from build123d import *

# Parameters (mm, degrees)
F1_W     = 12
F1_H     = 2
F3_R     = 10
F5_DEPTH = 12.001
F6_R     = 2.5
F7_DEPTH = 12.001
F8_R     = 5.99999
F9_R     = 5.99999


# Not quite as in the source:
# - a fillet or chamfer is up to 0.001 mm smaller than in the source, because OpenCascade refuses the exact size


with BuildPart() as f2:
    # F2: sweep along a path in F0
    with BuildLine(Plane.YZ) as f2_path:
        Line((0, 0), (20, 0))
        Line((20, 0), (35, 10))
        Line((35, 10), (92, 10))
    # F1 (on Front) → F2 (sweep)
    with BuildSketch(Plane.XZ):
        with Locations((0, 1)):
            Rectangle(F1_W, F1_H)
    sweep(path=f2_path.line, transition=Transition.RIGHT)

    # F3
    f3_edges = [f2.edges().sort_by_distance(p)[0] for p in [
        (0, 19.394449, 2),
        (0, 34.394449, 12),
        (0, 35, 10),
        (0, 20, 0),
    ]]
    fillet(f3_edges, radius=F3_R)

    # F4 (on Top) → F5 (cut, through all)
    with BuildSketch(Plane.XY):
        with BuildLine():
            Line((2, 4.5), (2, 7.5))
            ThreePointArc((2, 7.5), (0, 8.5), (-2, 7.5))
            Line((-2, 7.5), (-2, 4.5))
            ThreePointArc((-2, 4.5), (0, 3.5), (2, 4.5))
        make_face()
    extrude(amount=F5_DEPTH, mode=Mode.SUBTRACT)

    # F6 (on Top) → F7 (cut, through all)
    with BuildSketch(Plane.XY):
        with Locations((0, 86)):
            Circle(F6_R)
    extrude(amount=F7_DEPTH, mode=Mode.SUBTRACT)

    # F8 (radius 6 in the source; OpenCascade refuses exactly that, so slightly less here)
    f8_edges = [f2.edges().sort_by_distance(p)[0] for p in [
        (-6, 0, 1),
        (6, 0, 1),
    ]]
    fillet(f8_edges, radius=F8_R)

    # F9 (radius 6 in the source; OpenCascade refuses exactly that, so slightly less here)
    f9_edges = [f2.edges().sort_by_distance(p)[0] for p in [
        (6, 92, 11),
        (-6, 92, 11),
    ]]
    fillet(f9_edges, radius=F9_R)


solid = f2.part
Can you work these out from the model? Positions are in its coordinate system, mm. A direction names the side the tool comes from. Round coordinates to 2 decimals unless told otherwise and drop trailing zeros. Loops run counter-clockwise (first coordinate to the right, second up) from the corner with the lowest first, then second, coordinate; pieces in that order, holes last. Notation, with made-up numbers: (53, 23) - (77, 23) arc R11 ccw to (77, 33) - close; hole circle Ø11 at (41.25, 19.5). An arc over 180 degrees is marked (long way). Use CSV: the item, a comma, the result in double quotes. Start each with the question number.
1) For faces 5 (the flat face through (0, 65, 10)), 6 (the cylindrical face through (-0.084, 34.485, 11.559)), 7 (the cylindrical face through (0, 8.5, 1)), which set-ups out of +Z, -Z, +X, -X, +Y, -Y let a thin tool reach every point of the face, with its end or its side?
2) For pin 1 Ø1.5 at (x, y) = (-3, 32) entering from -Z, with a flat end and sliding along its axis, tell me the tip position at first contact or that it passes through.
3) If we section it at D-D on z = 5.25: Write out the boundary of the cut face in (x, y) (3 decimals), plus the area to 3 significant figures.
4) If we section it at C-C on y = 57: Write out the boundary of the cut face in (x, z).
5) If we section it at B-B on x = 4.5: Write out the boundary of the cut face in (y, z), plus the area to 3 significant figures.
6) If we section it at A-A on y = 84.5: Write out the boundary of the cut face in (x, z).
7) Please list where these lines run through material, in increasing order: probe 1 along X at (y, z) = (86, 10.6); probe 2 along Z at (x, y) = (-3.5, 61.5); probe 3 along Y at (x, z) = (0, 10.55). Write a range as [from, to].
8) We'd pull the mould along Y, two halves only. Please class faces 1 (the flat face through (0, 10, 2)), 2 (the cylindrical face through (0.08, 19.23, 2.42)), 3 (the cylindrical face through (-4.289, 90.196, 10.986)), 4 (the cylindrical face through (-0.33, 88.48, 10.99)): released by +Y, released by -Y, zero draft, split by the parting line, or undercut.
Geometry results:
1,face 5,"-Z, +X, -X, +Y"
1,face 6,"+Z, +X, -X, -Y"
1,face 7,"+Z, -Z"
2,pin 1,"stops at z = 7.5"
3,outline,"(-6, 24.269) - (6, 24.269) - (6, 27.875) - (-6, 27.875) - close"
3,area,"43.3 mm2"
4,outline,"(-6, 10) - (6, 10) - (6, 12) - (-6, 12) - close"
5,outline,"(2.03, 0) - (16.97, 0) arc R10 ccw to (22.52, 1.68) - (32.48, 8.32) arc R10 cw to (38.03, 10) - (89.97, 10) - (89.97, 12) - (37.42, 12) arc R10 ccw to (31.88, 10.32) - (21.91, 3.68) arc R10 cw to (16.37, 2) - (2.03, 2) - close"
5,area,"182 mm2"
6,outline,"(-6, 10) - (-2, 10) - (-2, 12) - (-6, 12) - close; (2, 10) - (6, 10) - (6, 12) - (2, 12) - close"
7,probe 1,"x = [-6, -2.5], [2.5, 6]"
7,probe 2,"z = [10, 12]"
7,probe 3,"y = [32.24, 83.5], [88.5, 92]"
8,face 1,"zero draft"
8,face 2,"released by -Y"
8,face 3,"released by +Y"
8,face 4,"undercut"
